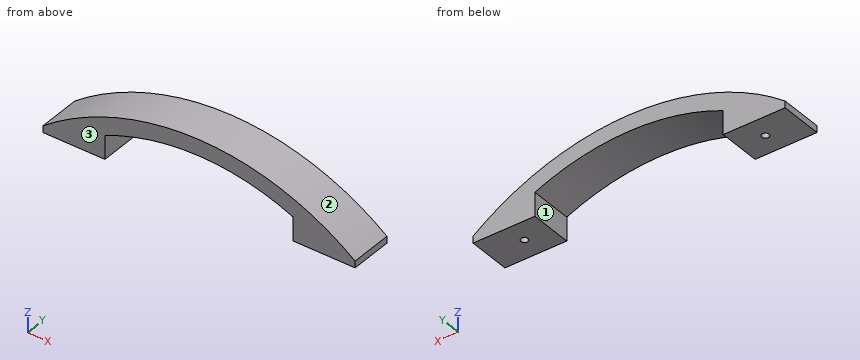
```python
from build123d import *

# Parameters (mm, degrees)
F2_DEPTH   = 8.509
F4_D       = 2.794
F4_DEPTH   = 7.62
F4_START   = 0.0673694
F4_START_2 = 0.0673774
F4_TIP     = 0.8394022848


with BuildPart() as f2:
    # F0 (on Front) → F2 (new body, symmetric)
    with BuildSketch(Plane.XZ):
        with BuildLine():
            ThreePointArc((55.7179713222, -8.0797821716), (-6.4739286778, 12.9986083689), (-68.6658286778, -8.0797821716))
            Line((-68.6658286778, -8.0797821716), (-68.6658286778, -10.7530225501))
            Line((-68.6658286778, -10.7530225501), (-44.0024286778, -10.7530225501))
            Line((-44.0024286778, -10.7530225501), (-44.0024286778, -1.3550225501))
            ThreePointArc((-44.0024286778, -1.3550225501), (-6.4739278287, 6.5894008462), (31.0545713222, -1.3550305716))
            Line((31.0545713222, -1.3550305716), (31.0545713222, -10.7530305716))
            Line((31.0545713222, -10.7530305716), (55.7179713222, -10.7530305716))
            Line((55.7179713222, -10.7530305716), (55.7179713222, -8.0797821716))
        make_face()
    extrude(amount=F2_DEPTH, both=True)


with BuildPart() as f2_1:
    # F3: moved
    add(f2.part.moved(Location((0, 0, 10.8204))))

    # F4
    # its depths count from where the whole tool has entered the part; down to there all is cleared
    with Locations(Plane(origin=(0, 0, 0), x_dir=(1, 0, 0), z_dir=(0, 0, -1))):
        with Locations((-54.4799286778, 0, -F4_START_2), (41.5204335099, 0, -F4_START)):
            Hole(F4_D / 2, depth=F4_DEPTH)
            with Locations((0, 0, -(F4_DEPTH + F4_TIP / 2))):  # 118° drill point
                Cone(0, F4_D / 2, F4_TIP, mode=Mode.SUBTRACT)


solid = f2_1.part
```
Geometry: final body of the model. Coordinates: model frame, mm. Face numbers are marked on the shaded views. Round coordinates to 2 decimals unless told otherwise and drop trailing zeros. Order: outer loops, then holes, each group sorted by start corner. A loop starts at its lowest first (then second) coordinate and runs counter-clockwise, first axis right, second up. Notation, with made-up numbers: M 36,-4.5 L 46,-4.5 A21 cw 46,8.5 Z; hole C 44.25,-18 d5. An arc over 180 degrees is marked long. Use one line per item in the form item = value. Start each with the question number.
Q1. Pin query (flat end, axial travel): pin 1 Ø4 at (x, z) = (-36, 9.5) entering from -Y; pin 2 Ø1.7 at (x, y) = (-54.48, 0) entering from +Z; pin 3 Ø4.5 at (y, z) = (-2.5, 3) entering from -X; pin 4 Ø8 at (x, y) = (-32.5, -6) entering from -Z. Return the tip coordinate at first contact, or that it passes through.
Q2. Material intervals for line 1 (X direction, y = 1.75, z = 8.25); line 2 (X direction, y = -7.5, z = 9.5); line 3 (Z direction, x = -28.5, y = 0), sorted ascending. Write a range as [from, to].
Q3. Cut plane B-B (z = 21.5). Return loops of the section in (x, y), and give its area (3 significant figures).
Q4. Cut plane C-C (x = -15). Return loops of the section in (y, z).
Q5. Mould query, pull axis X, two halves, no side actions, for the marked faces 1, 2 and 3. Classes: +X half, -X half, draft (parallel to the pull), parting line (faces both ways), or undercut.
Q6. Cut plane A-A (y = 6.25). Return loops of the section in (x, z).
Geometry results:
q1.pin_1 = through
q1.pin_2 = 12.3
q1.pin_3 = -68.67
q1.pin_4 = 12.41
q2.line_1 = [-60.72, -44], [31.05, 47.77]
q2.line_2 = [-58.67, -43.92], [30.98, 45.72]
q2.line_3 = [14.75, 21.42]
q3.outline = M -28.13,-8.51 L 15.18,-8.51 L 15.18,8.51 L -28.13,8.51 Z
q3.area = 737 mm^2
q4.outline = M -8.51,17.02 L 8.51,17.02 L 8.51,23.46 L -8.51,23.46 Z
q5.face_1 = undercut
q5.face_2 = parting line
q5.face_3 = draft
q6.outline = M -68.67,0.07 L -44,0.07 L -44,9.47 A92.61 cw 31.05,9.47 L 31.05,0.07 L 55.72,0.07 L 55.72,2.74 A102.29 ccw -68.67,2.74 Z
